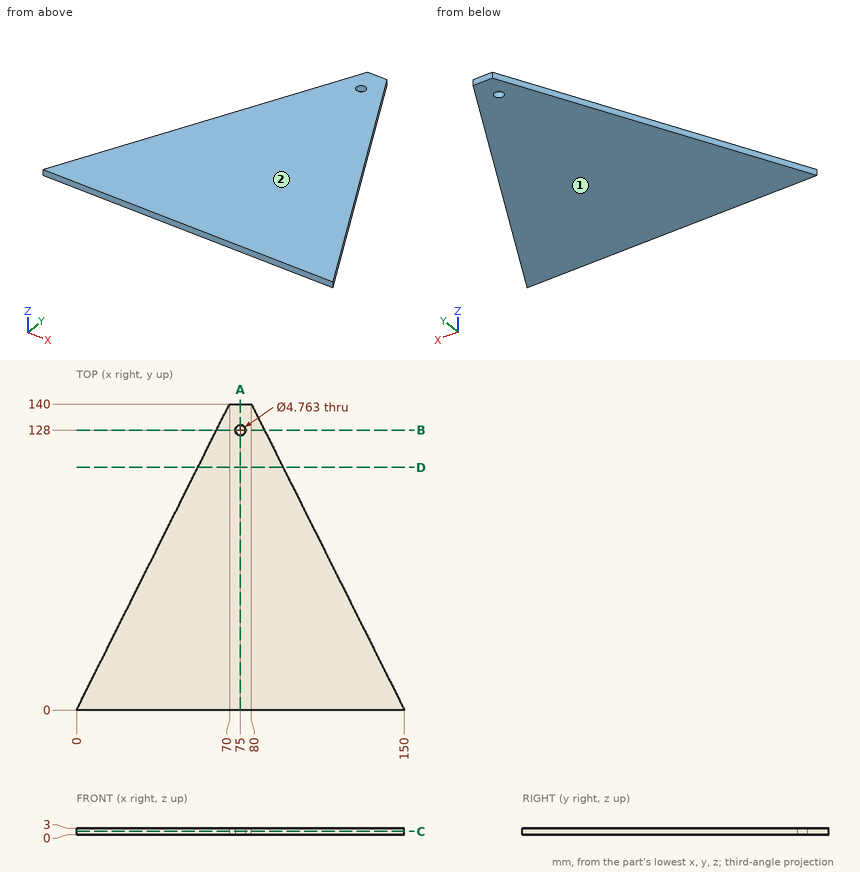
Part print with two shaded views. Sizes in mm from the minimum x, y, z corner. Coordinates: 2 decimals unless noted, no trailing zeros. Order: outer loops, then holes, each group sorted by start corner. A loop starts at its lowest first (then second) coordinate and runs counter-clockwise, first axis right, second up.
(1) Saw through at A-A, the plane x = 75. Write the cut outline in (y, z).
Solution:
outline: (0, 0) - (125.62, 0) - (125.62, 3) - (0, 3) - close; (130.38, 0) - (140, 0) - (140, 3) - (130.38, 3) - close
(2) Saw through at C-C, the plane z = 1.45. Write the cut outline in (x, y).
Solution:
outline: (0, 0) - (150, 0) - (80, 140) - (70, 140) - close; hole circle Ø4.76 at (75, 128)
(3) Saw through at B-B, the plane y = 128. Write the cut outline in (x, z).
Solution:
outline: (64, 0) - (72.62, 0) - (72.62, 3) - (64, 3) - close; (77.38, 0) - (86, 0) - (86, 3) - (77.38, 3) - close
(4) Drill centre lines: L1, parallel to Y at x = 75, z = 2.15; L2, parallel to X at y = 130, z = 0.4 (1 decimal); L3, parallel to Y at x = 134, z = 0.65 (1 decimal). Where is each one in solid material? Low to high.
Solution:
L1: y = 0 to 125.62, 130.38 to 140
L2: x = 65 to 73.7, 76.3 to 85
L3: y = 0 to 32
(5) Saw through at D-D, the plane y = 111. Write the cut outline in (x, z).
Solution:
outline: (55.5, 0) - (94.5, 0) - (94.5, 3) - (55.5, 3) - close
(6) Mould opens along Z. For the marked faces 1 and 2 say: released by +Z, released by -Z, zero draft, split by the parting line, or undercut.
Solution:
face 1: released by -Z
face 2: released by +Z
